Can you work these out from the model? Positions are in its coordinate system, mm. Give positions to 0.01 mm unless a question says otherwise; leave off trailing zeros. Write each loop counter-clockwise with the first axis right and the second up, starting at its lowest first coordinate (ties: lowest second). Pieces come first, ordered by that corner, then holes.
1. Thinking about a two-plate mould opening in X: for faces 1 (the cylindrical face through (-16.079, 5.07, 16.746)), 2 (the cylindrical face through (22.17, 4.93, 9.19)), which applies, pulls with the +X half, pulls with the -X half, needs draft (parallel to the pull), parting line crosses it, or undercut?
2. Suppose I cut it at C-C (x = 18). Please give me the cut outline in (y, z).
3. Suppose I cut it at B-B (z = 0). Please give me the cut outline in (x, y), and give its area (3 significant figures).
4. I'm going to push flat-ended pins straight in: pin 1 (5 mm diameter, centred on y = 1.5, z = -2.5, fed in from -X); pin 2 (1.2 mm diameter, centred on x = -18, y = 5.5, fed in from -Z); pin 3 (0.8 mm diameter, centred on x = 18, y = 7, fed in from +Z); pin 4 (17.5 mm diameter, centred on x = 0, z = 0, fed in from -Y). Where does each tip first touch, or does it pass through?
5. Suppose I cut it at D-D (y = 5). Give the number of separate pieces and of enclosed holes in the cut face, and give its area (3 significant figures).
6. Suppose I cut it at A-A (x = 0). Please give me the cut outline in (y, z) (3 decimals), and give its area (3 significant figures).
7. If I drill on probe 1 along Z at (x, y) = (0, 6.75) (3 decimals); probe 2 along Z at (x, y) = (11, 9); probe 3 along X at (y, z) = (3.5, -15.5), over which ranges is the centre line in solid material (lowest first)?
```python
from build123d import *

# Parameters (mm, degrees)
SKETCH3_R           = 24
SKETCH3_R_2         = 14.55
BOSS_EXTRUDE1_DEPTH = 10
CUT_EXTRUDE2_START  = 50
SKETCH4_R           = 2.5
CUT_EXTRUDE2_DEPTH  = 100
SKETCH5_R           = 1.5
CUT_EXTRUDE3_DEPTH  = 100
CUT_EXTRUDE6_DEPTH  = 26
CUT_EXTRUDE7_DEPTH  = 26
CUT_EXTRUDE8_DEPTH  = 26
CUT_EXTRUDE9_DEPTH  = 26
FILLET5_R           = 3


with BuildPart() as part:
    # Sketch3 → Boss-Extrude1 (new body)
    with BuildSketch(Plane(origin=(0, 0, 0), x_dir=(1, 0, 0), z_dir=(0, 1, 0))):
        Circle(SKETCH3_R)
        Circle(SKETCH3_R_2, mode=Mode.SUBTRACT)
    extrude(amount=BOSS_EXTRUDE1_DEPTH)

    # Sketch4 → Cut-Extrude2 (cut)
    with BuildSketch(Plane(origin=(0, 0, 0), x_dir=(0, 0, -1), z_dir=(1, 0, 0)).offset(CUT_EXTRUDE2_START)):
        with Locations((0, 5)):
            Circle(SKETCH4_R)
    extrude(amount=-CUT_EXTRUDE2_DEPTH, mode=Mode.SUBTRACT)

    # Sketch5 → Cut-Extrude3 (cut)
    with BuildSketch(Plane(origin=(0, 10, 0), x_dir=(1, 0, 0), z_dir=(0, 1, 0))):
        with Locations((0, 19.275)):
            Circle(SKETCH5_R)
        with Locations((0, -19.275)):
            Circle(SKETCH5_R)
    extrude(amount=-CUT_EXTRUDE3_DEPTH, mode=Mode.SUBTRACT)

    # Sketch7 → Cut-Extrude6 (cut)
    with BuildSketch(Plane(origin=(0, 10, 0), x_dir=(1, 0, 0), z_dir=(0, 1, 0))):
        with BuildLine():
            Line((3.5, 15.275), (3.5, 22.775))
            ThreePointArc((3.5, 22.775), (15.930450829, 16.648464235), (22.598686356, 4.5))
            Line((22.598686356, 4.5), (15.010850242, 4.5))
            ThreePointArc((15.010850242, 4.5), (10.709250694, 11.440610761), (3.5, 15.275))
        make_face()
    extrude(amount=-CUT_EXTRUDE6_DEPTH, mode=Mode.SUBTRACT)

    # Sketch9 → Cut-Extrude7 (cut)
    with BuildSketch(Plane(origin=(0, 10, 0), x_dir=(1, 0, 0), z_dir=(0, 1, 0))):
        with BuildLine():
            Line((15.010850242, -4.5), (22.775, -4.5))
            ThreePointArc((22.775, -4.5), (16.052855024, -16.770702746), (3.5, -22.94995915))
            Line((3.5, -22.94995915), (3.5, -15.275))
            ThreePointArc((3.5, -15.275), (10.709250694, -11.440610761), (15.010850242, -4.5))
        make_face()
    extrude(amount=-CUT_EXTRUDE7_DEPTH, mode=Mode.SUBTRACT)

    # Sketch10 → Cut-Extrude8 (cut)
    with BuildSketch(Plane(origin=(0, 10, 0), x_dir=(1, 0, 0), z_dir=(0, 1, 0))):
        with BuildLine():
            Line((-3.5, 15.275), (-3.5, 22.775))
            ThreePointArc((-3.5, 22.775), (-15.930450829, 16.648464235), (-22.598686356, 4.5))
            Line((-22.598686356, 4.5), (-15.010850242, 4.5))
            ThreePointArc((-15.010850242, 4.5), (-10.709250694, 11.440610761), (-3.5, 15.275))
        make_face()
    extrude(amount=-CUT_EXTRUDE8_DEPTH, mode=Mode.SUBTRACT)

    # Sketch11 → Cut-Extrude9 (cut)
    with BuildSketch(Plane(origin=(0, 10, 0), x_dir=(1, 0, 0), z_dir=(0, 1, 0))):
        with BuildLine():
            Line((-15.010850242, -4.5), (-22.775, -4.5))
            ThreePointArc((-22.775, -4.5), (-16.052855024, -16.770702746), (-3.5, -22.94995915))
            Line((-3.5, -22.94995915), (-3.5, -15.275))
            ThreePointArc((-3.5, -15.275), (-10.709250694, -11.440610761), (-15.010850242, -4.5))
        make_face()
    extrude(amount=-CUT_EXTRUDE9_DEPTH, mode=Mode.SUBTRACT)

    # Fillet5
    fillet5_edges = [part.edges().sort_by_distance(p)[0] for p in [
        (-3.5, 5, 22.94995915),
        (-22.775, 5, 4.5),
        (-15.010850242, 5, 4.5),
        (-3.5, 5, 15.275),
        (3.5, 5, -22.775),
        (22.598686356, 5, -4.5),
        (15.010850242, 5, -4.5),
        (3.5, 5, -15.275),
        (3.5, 5, 15.275),
        (15.010850242, 5, 4.5),
        (22.775, 5, 4.5),
        (3.5, 5, 22.94995915),
        (-3.5, 5, -15.275),
        (-15.010850242, 5, -4.5),
        (-22.598686356, 5, -4.5),
        (-3.5, 5, -22.775),
    ]]
    fillet(fillet5_edges, radius=FILLET5_R)


solid = part.part
```
Checks:
1. face 1: undercut
1. face 2: parting line crosses it
2. outline: (0, -15.87) - (10, -15.87) - (10, -14.39) - (0, -14.39) - close; (0, -4.5) - (10, -4.5) - (10, 4.5) - (0, 4.5) - close; (0, 14.66) - (10, 14.66) - (10, 15.87) - (0, 15.87) - close; hole circle Ø5 at (5, 0)
3. outline: (-24, 0) - (-14.55, 0) - (-14.55, 2.5) - (-24, 2.5) - close; (-24, 7.5) - (-14.55, 7.5) - (-14.55, 10) - (-24, 10) - close; (14.55, 0) - (24, 0) - (24, 2.5) - (14.55, 2.5) - close; (14.55, 7.5) - (24, 7.5) - (24, 10) - (14.55, 10) - close
3. area: 94.5 mm2
4. pin 1: stops at x = -24
4. pin 2: stops at z = -16.53
4. pin 3: stops at z = 16.32
4. pin 4: passes through
5. separate pieces: 2
5. enclosed holes: 6
5. area: 403 mm2
6. outline: (0, -24) - (10, -24) - (10, -20.775) - (0, -20.775) - close; (0, -17.775) - (10, -17.775) - (10, -14.55) - (0, -14.55) - close; (0, 14.55) - (10, 14.55) - (10, 17.775) - (0, 17.775) - close; (0, 20.775) - (10, 20.775) - (10, 24) - (0, 24) - close
6. area: 129 mm2
7. probe 1: z = -24 to -20.775, -17.775 to -14.55, 14.55 to 17.775, 20.775 to 24
7. probe 2: z = -21.33 to -20.25, -11.16 to -9.52, 9.52 to 11.16, 20.44 to 21.33
7. probe 3: x = -18.32 to -17.05, -4.27 to 4.27, 17.05 to 18.32
